Verification items for this drawing (mm, ordinates from the low corner). Coordinates: 2 decimals unless noted, no trailing zeros. Loops run counter-clockwise (first coordinate to the right, second up) from the corner with the lowest first, then second, coordinate; pieces in that order, holes last. Notation, with made-up numbers: M 62,18 L 103,18 A31 ccw 103,47 Z; hole C 53.5,15.25 d4. An arc over 180 degrees is marked long. Return JSON: item names as keys, results as strings.
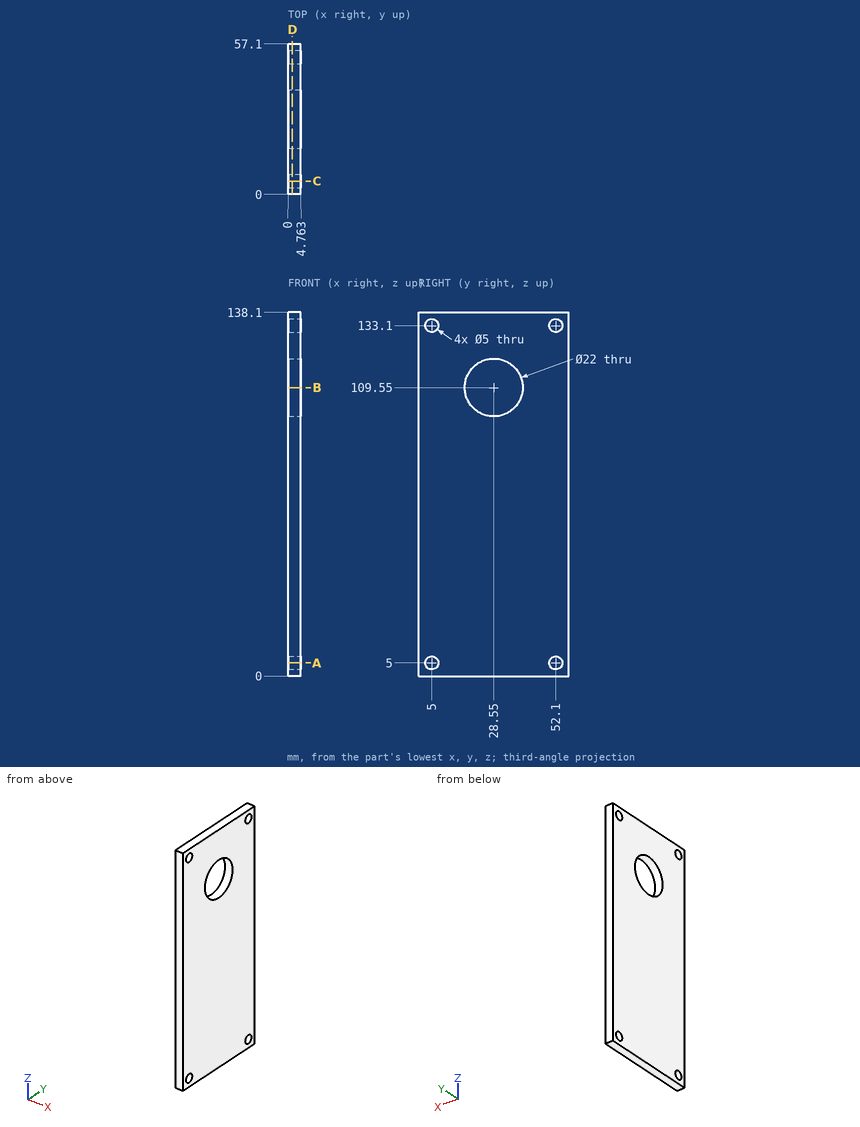
1) Go/stop test with flat-tipped pins: pin 1 Ø3 at (y, z) = (5, 5) entering from +X; pin 2 Ø6 at (y, z) = (18.5, 14) entering from -X. Record where each tip stops, or that it passes through.
Answers:
{"pin 1": "through", "pin 2": "x = 0"}
2) Section check D-D on x = 1.6. Record the cut outline in (y, z).
Answers:
{"outline": "M 0,0 L 57.1,0 L 57.1,138.1 L 0,138.1 Z; hole C 5,5 d5; hole C 5,133.1 d5; hole C 28.55,109.55 d22; hole C 52.1,5 d5; hole C 52.1,133.1 d5"}
3) Section check B-B on z = 109.55. Record the cut outline in (x, y).
Answers:
{"outline": "M 0,0 L 4.76,0 L 4.76,17.55 L 0,17.55 Z; M 0,39.55 L 4.76,39.55 L 4.76,57.1 L 0,57.1 Z"}
4) Section check A-A on z = 5. Record the cut outline in (x, y).
Answers:
{"outline": "M 0,0 L 4.76,0 L 4.76,2.5 L 0,2.5 Z; M 0,7.5 L 4.76,7.5 L 4.76,49.6 L 0,49.6 Z; M 0,54.6 L 4.76,54.6 L 4.76,57.1 L 0,57.1 Z"}
5) Section check C-C on y = 5. Record the cut outline in (x, z).
Answers:
{"outline": "M 0,0 L 4.76,0 L 4.76,2.5 L 0,2.5 Z; M 0,7.5 L 4.76,7.5 L 4.76,130.6 L 0,130.6 Z; M 0,135.6 L 4.76,135.6 L 4.76,138.1 L 0,138.1 Z"}
6) Scan lines: line 1 along Z through (x, y) = (1.5, 52.1); line 2 along Z through (x, y) = (0.8, 29); line 3 along Y through (x, z) = (1.9, 109.55). Record each from-to range of solid material in increasing order. Write a range as [from, to].
Answers:
{"line 1": "[0, 2.5], [7.5, 130.6], [135.6, 138.1]", "line 2": "[0, 98.56], [120.54, 138.1]", "line 3": "[0, 17.55], [39.55, 57.1]"}
